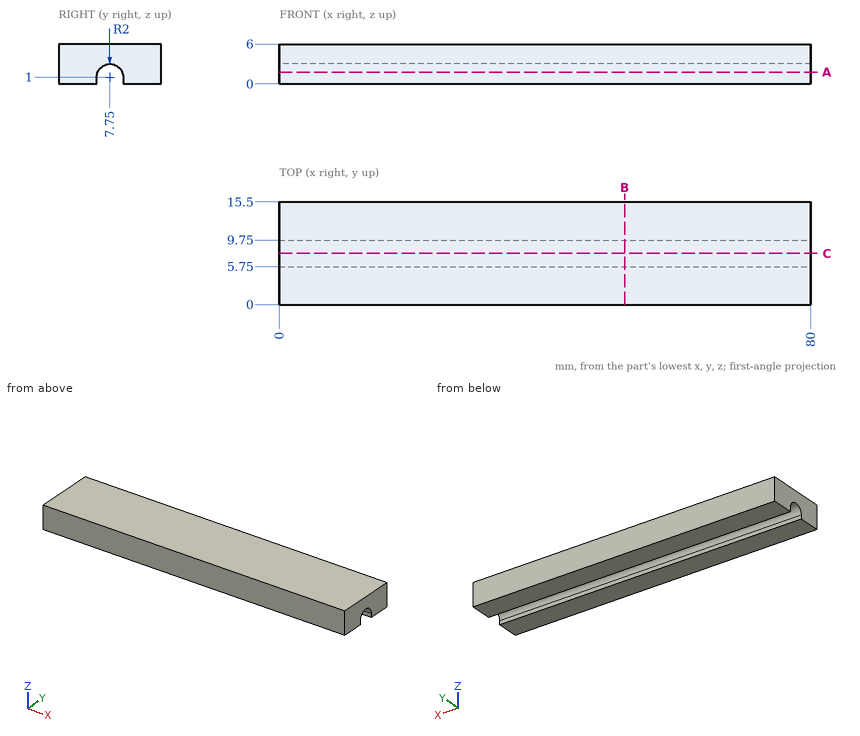
Can you work these out from the drawing? Everything is in mm from the part's minimum corner. Round coordinates to 2 decimals unless told otherwise and drop trailing zeros. Loops run counter-clockwise (first coordinate to the right, second up) from the corner with the lowest first, then second, coordinate; pieces in that order, holes last. Notation, with made-up numbers: (-34.5, -21) -> (13.5, -21) arc R11 ccw to (13.5, -7) -> close; hole circle Ø4 at (-16.75, 52). An arc over 180 degrees is marked (long way). Use CSV: the item, a comma, the result in double quotes.
(1) Will this pin go through, and if not, where does the flat tip stop? pin 1 Ø3 at (x, y) = (59, 10.5) entering from -Z.
Return value:
pin 1,"stops at z = 0"
(2) Suppose I cut it at A-A on z = 1.75. Write out the boundary of the cut face in (x, y), plus the area to 3 significant figures.
Return value:
outline,"(0, 0) -> (80, 0) -> (80, 5.9) -> (0, 5.9) -> close; (0, 9.6) -> (80, 9.6) -> (80, 15.5) -> (0, 15.5) -> close"
area,"943 mm²"
(3) If I drill on probe 1 along Y at (x, z) = (49, 1.05); probe 2 along Z at (x, y) = (27, 6.75), over which ranges is the centre line in solid material (lowest first)? Write a range as [from, to].
Return value:
probe 1,"y = [0, 5.75], [9.75, 15.5]"
probe 2,"z = [2.73, 6]"
(4) Suppose I cut it at B-B on x = 52. Write out the boundary of the cut face in (y, z).
Return value:
outline,"(0, 0) -> (5.75, 0) -> (5.75, 1) arc R2 cw to (9.75, 1) -> (9.75, 0) -> (15.5, 0) -> (15.5, 6) -> (0, 6) -> close"
(5) Suppose I cut it at C-C on y = 7.75. Write out the boundary of the cut face in (x, z), plus the area to 3 significant figures.
Return value:
outline,"(0, 3) -> (80, 3) -> (80, 6) -> (0, 6) -> close"
area,"240 mm²"
